```python
from build123d import *

# Parameters (mm, degrees)
F1_DEPTH = 100


with BuildPart() as f1:
    # F0 (on Front) → F1 (new body)
    with BuildSketch(Plane.XZ):
        with BuildLine():
            Line((0, 85), (0, 0))
            Line((0, 0), (12.5, 0))
            Line((12.5, 0), (12.5, 3))
            ThreePointArc((12.5, 3), (11.914214, 4.414214), (10.5, 5))
            Line((10.5, 5), (5, 5))
            ThreePointArc((5, 5), (3.585786, 5.585786), (3, 7))
            Line((3, 7), (3, 27))
            ThreePointArc((3, 27), (3.585786, 28.414214), (5, 29))
            Line((5, 29), (5, 66.111684))
            ThreePointArc((5, 66.111684), (5.861427, 67.755963), (7.703652, 67.983815))
            Line((7.703652, 67.983815), (128.938041, 22.417103))
            ThreePointArc((128.938041, 22.417103), (130.100091, 21.794695), (131.05909, 20.89022))
            Line((131.05909, 20.89022), (154.73982, -8.247924))
            ThreePointArc((154.73982, -8.247924), (155.698819, -9.152399), (156.86087, -9.774807))
            Line((156.86087, -9.774807), (182.2, -19.29868))
            ThreePointArc((182.2, -19.29868), (181.585124, -15.998362), (179.021539, -13.830829))
            Line((179.021539, -13.830829), (159.281959, -6.411583))
            ThreePointArc((159.281959, -6.411583), (158.119909, -5.789175), (157.16091, -4.8847))
            Line((157.16091, -4.8847), (133.48018, 24.253443))
            ThreePointArc((133.48018, 24.253443), (132.521181, 25.157918), (131.35913, 25.780327))
            Line((131.35913, 25.780327), (10.481739, 71.212859))
            ThreePointArc((10.481739, 71.212859), (5.778607, 74.88065), (4, 80.573513))
            Line((4, 80.573513), (4, 81))
            ThreePointArc((4, 81), (2.828427, 83.828427), (0, 85))
        make_face()
    extrude(amount=F1_DEPTH)


solid = f1.part
```
Work out the finished part from the listing and answer in its coordinate system (mm). A direction names the side the tool comes from. Round coordinates to 2 decimals unless told otherwise and drop trailing zeros. Loops run counter-clockwise (first coordinate to the right, second up) from the corner with the lowest first, then second, coordinate; pieces in that order, holes last. Notation, with made-up numbers: M 7,71 L 41,71 A26 ccw 41,86 Z; hole C 61.25,76.25 d1. An arc over 180 degrees is marked long. One line per question, with ' | ' between items.
Q1. Find section B-B, the plane y = -36. Give the vertices of the cut face in (x, z).
Conclusion:
outline: M 0,0 L 12.5,0 L 12.5,3 A2 ccw 10.5,5 L 5,5 A2 cw 3,7 L 3,27 A2 cw 5,29 L 5,66.11 A2 cw 7.7,67.98 L 128.94,22.42 A5 cw 131.06,20.89 L 154.74,-8.25 A5 ccw 156.86,-9.77 L 182.2,-19.3 A5 ccw 179.02,-13.83 L 159.28,-6.41 A5 cw 157.16,-4.88 L 133.48,24.25 A5 ccw 131.36,25.78 L 10.48,71.21 A10 cw 4,80.57 L 4,81 A4 ccw 0,85 Z
Q2. Find section D-D, the plane x = 152. Give the vertices of the cut face in (y, z).
Conclusion:
outline: M -100,-4.88 L 0,-4.88 L 0,1.47 L -100,1.47 Z
Q3. Consider line 1 along X through (y, z) = (-84, 15); line 2 along Z through (x, y) = (9.5, -71.5); line 3 along X through (y, z) = (-75.5, 7.5). Determine where each line is inside the solid, lowest interval first. Write a range as from..to.
Conclusion:
line 1: x = 0..3, 135.85..141 | line 2: z = 0..5, 67.31..71.64 | line 3: x = 0..3, 141.94..147.1
Q4. Each of these flat-tipped pins is pushed along its axis until it touches: pin 1 Ø5 at (y, z) = (-55.5, 20) entering from +X; pin 2 Ø3 at (x, y) = (8, -74) entering from +Z; pin 3 Ø10 at (x, y) = (7.5, -39.5) entering from -Z. Where does it stop, or does it pass through?
Conclusion:
pin 1: stops at x = 138.97 | pin 2: stops at z = 73.96 | pin 3: stops at z = 0
Q5. The mould has two halves that part along Z. Classify faces 5 (the flat face through (3, -49, 17)), 6 (the flat face through (64, -100, 49)), 7 (the flat face through (145.486, -49.3, 9.48)), 8 (the flat face through (5, -49, 47)): +Z half, -Z half, draft (parallel to the pull), parting line (faces both ways), or undercut.
Conclusion:
face 5: undercut | face 6: draft | face 7: +Z half | face 8: undercut
Q6. Find section A-A, the plane z = 41. Give the vertices of the cut face in (x, y), then the cut area to 3 significant figures.
Conclusion:
outline: M 0,-100 L 5,-100 L 5,0 L 0,0 Z; M 79.5,-100 L 90.87,-100 L 90.87,0 L 79.5,0 Z | area: 1,640 mm2
Q7. A tool of negligible diameter and unlimited length cuts with its end or side. For faces 1 (the flat face through (142.73, -49.3, 6.53)), 2 (the flat face through (6, -49, 0)), 3 (the flat face through (8, -49, 5)), 4 (the flat face through (64, 0, 49)), from which of +Z, -Z, +X, -X, +Y, -Y can it reach the whole face along a straight path? Write none if from no direction.
Conclusion:
face 1: -Z, +Y, -Y | face 2: -Z, -X, +Y, -Y | face 3: +Y, -Y | face 4: +Z, -Z, +X, -X, +Y
Q8. Find section C-C, the plane z = 18.5. Give the vertices of the cut face in (x, y), then the cut area to 3 significant figures.
Conclusion:
outline: M 0,-100 L 3,-100 L 3,0 L 0,0 Z; M 133,-100 L 138.16,-100 L 138.16,0 L 133,0 Z | area: 815 mm2
